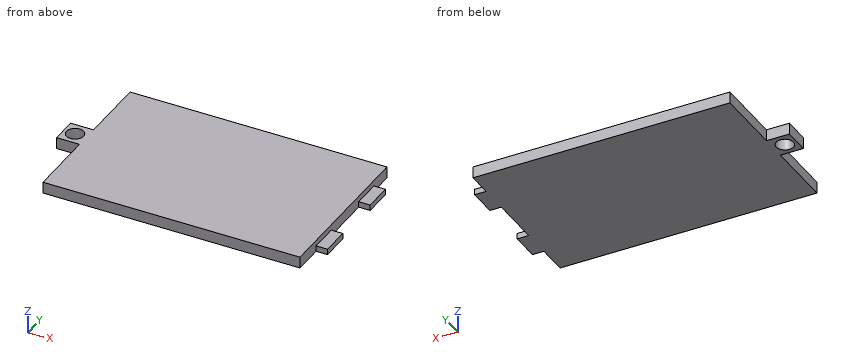
```python
from build123d import *

# Parameters (mm, degrees)
PAD003_DEPTH    = 2
SKETCH011_R     = 1.5
POCKET007_DEPTH = 5
SKETCH012_W     = 5
SKETCH012_H     = 1
PAD004_DEPTH    = 2


with BuildPart() as part:
    # Sketch010 → Pad003 (new body)
    with BuildSketch(Plane.XY.offset(25)):
        Polygon((-16, 25.8), (28.8, 25.8), (28.8, -2.8), (-16, -2.8), (-16, 9.2), (-20, 9.2), (-20, 13.8), (-16, 13.8), align=None)
    extrude(amount=PAD003_DEPTH)

    # Sketch011 (on Face10 of Pad003) → Pocket007 (cut)
    with BuildSketch(Plane.XY.offset(27)):
        with Locations((-18, 11.5)):
            Circle(SKETCH011_R)
    extrude(amount=-POCKET007_DEPTH, mode=Mode.SUBTRACT)

    # Sketch012 (on Face3 of Pocket007) → Pad004 (join)
    with BuildSketch(Plane.YZ.offset(28.8)):
        with Locations((5, 25.5)):
            Rectangle(SKETCH012_W, SKETCH012_H)
        with Locations((19, 25.5)):
            Rectangle(SKETCH012_W, SKETCH012_H)
    extrude(amount=PAD004_DEPTH)


solid = part.part
```
Source: CAD feature listing. Evaluate the final solid. Frame: model axes, mm. Coordinates: 2 decimals unless noted, no trailing zeros. Loops run counter-clockwise (first coordinate to the right, second up) from the corner with the lowest first, then second, coordinate; pieces in that order, holes last. Notation, with made-up numbers: M -11,-33 L 4,-33 A15 cw 4,-27 Z; hole C 72.25,68 d10. An arc over 180 degrees is marked long. Use a Markdown table: item, result. Add a question column.
Q1. Section query C-C, the plane x = -18. Return loops of the section in (y, z).
Q2. Section query B-B, the plane z = 25.55. Return loops of the section in (x, y).
Q3. First-contact query: pin 1 (0.8 mm diameter, centred on x = 29.5, z = 25.5, fed in from -Y); pin 2 (0.5 mm diameter, centred on x = 29.5, z = 25.5, fed in from +Y); pin 3 (0.6 mm diameter, centred on x = 30, y = 18, fed in from +Z); pin 4 (5 mm diameter, centred on x = -18, y = 11.5, fed in from +Z). Flat tips, straight axial feed; report the tip coordinate or a pass-through.
Q4. Section query A-A, the plane y = 11.5. Return loops of the section in (x, z), and give its area (3 significant figures).
Q5. Section query D-D, the plane y = 3. Return loops of the section in (x, z), and give its area (3 significant figures).
Q6. Material intervals for L1, parallel to Y at x = -18, z = 25.7; L2, parallel to X at y = 22.75, z = 25.35; L3, parallel to X at y = 6, z = 25.3, sorted ascending.
Result:
| question | item | result |
|---|---|---|
| 1 | outline | M 9.2,25 L 10,25 L 10,27 L 9.2,27 Z; M 13,25 L 13.8,25 L 13.8,27 L 13,27 Z |
| 2 | outline | M -20,9.2 L -16,9.2 L -16,-2.8 L 28.8,-2.8 L 28.8,2.5 L 30.8,2.5 L 30.8,7.5 L 28.8,7.5 L 28.8,16.5 L 30.8,16.5 L 30.8,21.5 L 28.8,21.5 L 28.8,25.8 L -16,25.8 L -16,13.8 L -20,13.8 Z; hole C -18,11.5 d3 |
| 3 | pin 1 | stops at y = 2.5 |
| 3 | pin 2 | stops at y = 21.5 |
| 3 | pin 3 | stops at z = 26 |
| 3 | pin 4 | stops at z = 27 |
| 4 | outline | M -20,25 L -19.5,25 L -19.5,27 L -20,27 Z; M -16.5,25 L 28.8,25 L 28.8,27 L -16.5,27 Z |
| 4 | area | 91.6 mm2 |
| 5 | outline | M -16,25 L 30.8,25 L 30.8,26 L 28.8,26 L 28.8,27 L -16,27 Z |
| 5 | area | 91.6 mm2 |
| 6 | L1 | y = 9.2 to 10, 13 to 13.8 |
| 6 | L2 | x = -16 to 28.8 |
| 6 | L3 | x = -16 to 30.8 |
